Work out the finished part from the listing and answer in its coordinate system (mm). A direction names the side the tool comes from. Coordinates: 2 decimals unless noted, no trailing zeros. Write each loop counter-clockwise with the first axis right and the second up, starting at its lowest first coordinate (ties: lowest second). Pieces come first, ordered by that corner, then holes. Notation, with made-up numbers: M 78.5,43 L 123.5,43 A12 ccw 123.5,48 Z; hole C -38.75,-15 d9. An arc over 180 degrees is marked long. Answer as CSV lines item,"result". Start each with the question number.
(1) Find the intervals of material crossed by L1, parallel to X at y = 1.45, z = -70; L2, parallel to X at y = 3.4, z = -9; L3, parallel to Z at x = -18.2, y = 2.75, in increasing order. Write a range as [from, to].
(2) A cutting plane is placed at D-D on y = 0.8. Count the separate pieces of the cut face and the enclosed holes in it, then the cut area to 3 significant figures.
(3) A cutting plane is placed at A-A on x = 5. Give the vertices of the cut face in (y, z), then the cut area to 3 significant figures.
(4) A flat-ended cylindrical pin translates along its axis: P1, Ø1.8, axis at x = 19.18, z = -2.4, coming from the +Y side. Find the tip coordinate at first contact, or state that the pin passes through.
(5) A cutting plane is placed at B-B on z = -15.3. Give the vertices of the cut face in (x, y), then the cut area to 3 significant figures.
(6) The mould has two halves that part along Z. Classify faces 1 (the cylindrical face through (29.2, 2.54, -74.16)), 2 (the flat face through (21.5, 2, -26)), 3 (the flat face through (0, 0, 1)): released by +Z, released by -Z, zero draft, split by the parting line, or undercut.
(7) For faces 4 (the flat face through (-21.5, 2, -26)), 5 (the flat face through (0, 2, 75)), determine the directions among +Z, -Z, +X, -X, +Y, -Y from which every point of the face is accessible in a straight line to the end or side of a thin tool.
(8) A cutting plane is placed at C-C on z = 70. Give the vertices of the cut face in (x, y).
Autodesk Inventor part; units mm, degrees
ref_plane "YZ Plane" through (0, 0, 0) normal (1, 0, 0) x (0, 1, 0)
ref_plane "XZ Plane" through (0, 0, 0) normal (0, 1, 0) x (-1, 0, 0)
ref_plane "XY Plane" through (0, 0, 0) normal (0, 0, 1) x (1, 0, 0)
sketch "Sketch1" plane through (0, 0, 0) normal (0, 1, 0) x (-1, 0, 0)
  line L0 (-30, 75) -> (30, 75)
  line L1 (30, 75) -> (30, -75)
  line L2 (30, -75) -> (-30, -75)
  line L3 (-30, -75) -> (-30, 75)
  line L4 (-30, 75) -> (30, -75) construction
  line L5 (30, 75) -> (-30, -75) construction
  line L6 (30, 75) -> (25, 75)
  line L7 (25, 75) -> (25, 70)
  line L8 (25, 70) -> (30, 70)
  line L9 (30, 70) -> (30, 75)
  line L10 (-30, 75) -> (-25, 75)
  line L11 (-25, 75) -> (-25, 70)
  line L12 (-25, 70) -> (-30, 70)
  line L13 (-30, 70) -> (-30, 75)
  line L14 (30, -75) -> (25, -75)
  line L15 (25, -75) -> (25, -70)
  line L16 (25, -70) -> (30, -70)
  line L17 (30, -70) -> (30, -75)
  line L18 (-30, -75) -> (-25, -75)
  line L19 (-25, -75) -> (-25, -70)
  line L20 (-25, -70) -> (-30, -70)
  line L21 (-30, -70) -> (-30, -75)
  circle A0 centre (25, 70) radius 1.4
  circle A1 centre (-25, 70) radius 1.4
  circle A2 centre (25, -70) radius 1.4
  circle A3 centre (-25, -70) radius 1.4
  line L22 (30, -75) -> (-30, -75)
  line L23 (-30, -75) -> (-30, -55)
  line L24 (-30, -55) -> (30, -55)
  line L25 (30, -55) -> (30, -75)
  line L26 (0, -55) -> (21.5, -55)
  line L27 (21.5, -55) -> (21.5, -12)
  line L28 (21.5, -12) -> (0, -12)
  line L29 (0, -12) -> (0, -55)
  line L30 (0, -12) -> (-21.5, -12)
  line L31 (-21.5, -12) -> (-21.5, -55)
  line L32 (-21.5, -55) -> (0, -55)
  line L33 (0, -55) -> (0, -12)
  line L34 (0, -12) -> (0, -33.5)
  line L35 (-18.2, -15.3) -> (18.2, -15.3)
  line L36 (18.2, -15.3) -> (18.2, -51.7)
  line L37 (18.2, -51.7) -> (-18.2, -51.7)
  line L38 (-18.2, -51.7) -> (-18.2, -15.3)
  line L39 (-18.2, -15.3) -> (18.2, -51.7) construction
  line L40 (18.2, -15.3) -> (-18.2, -51.7) construction
  circle A4 centre (18.2, -15.3) radius 1.5
  circle A5 centre (18.2, -51.7) radius 1.5
  circle A6 centre (-18.2, -15.3) radius 1.5
  circle A7 centre (-18.2, -51.7) radius 1.5
  line L41 (-30, 75) -> (-19.18, 75)
  line L42 (-19.18, 75) -> (-19.18, -2.4)
  line L43 (-19.18, -2.4) -> (-30, -2.4)
  line L44 (-30, -2.4) -> (-30, 75)
  line L45 (30, 75) -> (24, 75)
  line L46 (24, 75) -> (24, 48.4)
  line L47 (24, 48.4) -> (30, 48.4)
  line L48 (30, 48.4) -> (30, 75)
  circle A8 centre (24, 48.4) radius 1.5
  circle A9 centre (-19.18, -2.4) radius 1.5
  line L49 (-21.5, -12) -> (-21.5, -22)
  line L50 (-21.5, -22) -> (-25.5, -22)
  line L51 (-25.5, -22) -> (-25.5, -30)
  line L52 (-25.5, -30) -> (-21.5, -30)
  line L53 (-21.5, -30) -> (-21.5, -22)
  line L54 (21.5, -22) -> (25.5, -22)
  line L55 (25.5, -22) -> (25.5, -30)
  line L56 (25.5, -30) -> (21.5, -30)
  line L57 (21.5, -30) -> (21.5, -22)
  line L58 (21.5, -12) -> (15.5, -12)
  line L59 (15.5, -12) -> (5.5, -12)
  line L60 (5.5, -12) -> (5.5, -8)
  line L61 (5.5, -8) -> (15.5, -8)
  line L62 (15.5, -8) -> (15.5, -12)
  line L63 (-21.5, -12) -> (-16.5, -12)
  line L64 (-16.5, -12) -> (-0.5, -12)
  line L65 (-0.5, -12) -> (-0.5, -8)
  line L66 (-0.5, -8) -> (-16.5, -8)
  line L67 (-16.5, -8) -> (-16.5, -12)
  line L68 (21.5, -12) -> (10.5, -12)
  line L69 (10.5, -12) -> (10.5, -2.4)
  line L70 (10.5, -2.4) -> (21.5, -2.4)
  line L71 (21.5, -2.4) -> (21.5, -12)
  line L72 (5.5, -8) -> (10.5, -2.4)
  point P0 (10.5, -8)
  dimension "d10" = 60
  dimension "d11" = 150
  dimension "d12" = 5
  dimension "d13" = 5
  dimension "d14" = 5
  dimension "d15" = 5
  dimension "d16" = 5
  dimension "d17" = 5
  dimension "d18" = 5
  dimension "d19" = 5
  dimension "d20" = 2.8
  dimension "d21" = 2.8
  dimension "d22" = 2.8
  dimension "d23" = 2.8
  dimension "d28" = 20
  dimension "d29" = 21.5
  dimension "d30" = 43
  dimension "d31" = 21.5
  dimension "d32" = 36.4
  dimension "d33" = 36.4
  dimension "d34" = 3
  dimension "d35" = 3
  dimension "d36" = 3
  dimension "d37" = 3
  dimension "d38" = 10.82
  dimension "d39" = 77.4
  dimension "d40" = 6
  dimension "d41" = 26.6
  dimension "d42" = 3
  dimension "d43" = 3
  dimension "d48" = 10
  dimension "d49" = 4
  dimension "d50" = 8
  dimension "d51" = 4
  dimension "d52" = 8
  dimension "d53" = 6
  dimension "d54" = 10
  dimension "d55" = 4
  dimension "d56" = 5
  dimension "d57" = 16
  dimension "d58" = 4
extrude "Extrusion1" add sketch "Sketch1" along normal blind 5 contours L0 L11 A1 L12 L3 | L0 L42 A9 L43 L3 L12 A1 L11 | L0 L46 A0 A8 L47 L1 L24 L27 L56 L55 L54 L71 L70 L72 L60 L28 L30 L65 L66 L67 L31 L50 L51 L52 L3 L43 A9 L42 | L0 L7 A0 L46 | A9 L43 L42 | L42 L43 A9 | L24 L1 L16 A2 L15 L2 L19 A3 L20 L3 | L0 L1 L8 A0 L7 | L20 A3 L19 L2 L3 | L31 L30 L29 L35 A6 L38 A7 L37 L24 | A0 L8 L1 L47 A8 L46 | L29 L37 A5 L36 A4 L35 L28 L27 L24 | L52 L51 L50 L31 | A8 L47 L46 | L46 L47 A8 | L37 A7 L38 A6 L35 L29 | L29 L35 A4 L36 A5 L37 | L15 A2 L16 L1 L2 | L27 L54 L55 L56 | A5 L36 L37 | L37 L36 A5 | A7 L38 L37 | L37 L38 A7 | L67 L66 L65 L30 | L28 L62 L61 L69 L70 L71 | A6 L38 L35 | L35 L38 A6 | A4 L36 L35 | L35 L36 A4 | L28 L69 L61 L62 | L60 L61 L69 L28 | L69 L61 L72
fillet "Fillet1" radius 2.8 1 edges at (30, 2.5, 75)
fillet "Fillet2" radius 2.8 3 edges at (-30, 2.5, 75) (-30, 2.5, -75) (30, 2.5, -75)
extrude "Extrusion2" cut sketch "Sketch1" along normal blind 10 contours A8 L47 L46 | L46 L47 A8 | A5 L36 L37 | L37 L36 A5 | A7 L38 L37 | L37 L38 A7 | A6 L38 L35 | L35 L38 A6 | A4 L36 L35 | L35 L36 A4
extrude "Extrusion3" cut sketch "Sketch1" along normal blind 10 contours A9 L43 L42 | L42 L43 A9
extrude "Extrusion4" cut sketch "Sketch1" along normal blind 10 contours L52 L51 L50 L31 | L27 L54 L55 L56 | L67 L66 L65 L30 | L28 L69 L61 L62 | L60 L61 L69 L28
extrude "Extrusion5" cut sketch "Sketch1" along normal blind 10 contours L28 L62 L61 L69 L70 L71
extrude "Extrusion6" cut sketch "Sketch1" along normal blind 10 contours L69 L61 L72
fillet "Fillet3" radius 1 17 edges at (-5.5, 2.5, -8) (-10.5, 2.5, -2.4) (-21.5, 2.5, -2.4) (-21.5, 2.5, -12) (-5.5, 2.5, -12) (0.5, 2.5, -8) (0.5, 2.5, -12) (16.5, 2.5, -12) (16.5, 2.5, -8) (25.5, 2.5, -22) (21.5, 2.5, -22) (25.5, 2.5, -30) (21.5, 2.5, -30) (-25.5, 2.5, -30) (-25.5, 2.5, -22) (-21.5, 2.5, -22) (-21.5, 2.5, -30)
properties part number "DeGiua"
Here are the results:
1,L1,"x = [-30, -26.4], [-23.6, 23.6], [26.4, 30]"
1,L2,"x = [-30, -21.5], [-5.5, 0.5], [16.5, 30]"
1,L3,"z = [-75, -53.2], [-50.2, -16.8], [-13.8, -12], [-2.4, 75]"
2,separate pieces,"1"
2,enclosed holes,"14"
2,area,"8,660 mm^2"
3,outline,"M 0,-75 L 5,-75 L 5,-12 L 0,-12 Z; M 0,-8 L 5,-8 L 5,75 L 0,75 Z"
3,area,"730 mm^2"
4,P1,"passes through"
5,outline,"M -30,0 L -19.7,0 L -19.7,5 L -30,5 Z; M -16.7,0 L 16.7,0 L 16.7,5 L -16.7,5 Z; M 19.7,0 L 30,0 L 30,5 L 19.7,5 Z"
5,area,"270 mm^2"
6,face 1,"released by -Z"
6,face 2,"undercut"
6,face 3,"zero draft"
7,face 4,"+Y, -Y"
7,face 5,"+Z, +X, -X, +Y, -Y"
8,outline,"M -30,0 L -26.4,0 L -26.4,5 L -30,5 Z; M -23.6,0 L 23.6,0 L 23.6,5 L -23.6,5 Z; M 26.4,0 L 30,0 L 30,5 L 26.4,5 Z"
